from build123d import *

# Parameters (mm, degrees)
CROQUIS1_W              = 44
CROQUIS1_H              = 20
CROQUIS1_R              = 8
SALIENTE_EXTRUIR1_DEPTH = 15
CROQUIS2_R              = 1.75
CORTAR_EXTRUIR1_DEPTH   = 22


with BuildPart() as part:
    # Croquis1 → Saliente-Extruir1 (new body)
    with BuildSketch(Plane.XY):
        Rectangle(CROQUIS1_W, CROQUIS1_H)
        with Locations((-11, 0)):
            Circle(CROQUIS1_R, mode=Mode.SUBTRACT)
        with Locations((11, 0)):
            Circle(CROQUIS1_R, mode=Mode.SUBTRACT)
    extrude(amount=SALIENTE_EXTRUIR1_DEPTH)

    # Croquis2 → Cortar-Extruir1 (cut)
    with BuildSketch(Plane.XY.offset(15)):
        with Locations((-19, 7)):
            Circle(CROQUIS2_R)
        with Locations((19, -7)):
            Circle(CROQUIS2_R)
        with Locations((19, 7)):
            Circle(CROQUIS2_R)
        with Locations((-19, -7)):
            Circle(CROQUIS2_R)
    extrude(amount=-CORTAR_EXTRUIR1_DEPTH, mode=Mode.SUBTRACT)


solid = part.part
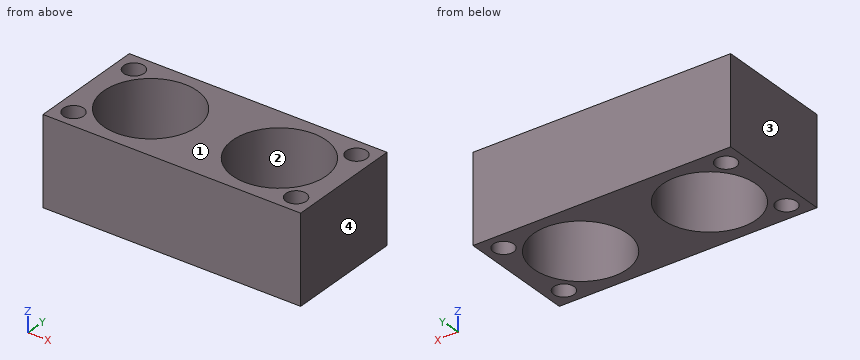
Here's how the part is built. I have some questions about the finished solid (model axes, mm). Face numbers are marked on the shaded views. Coordinates: 2 decimals unless noted, no trailing zeros. Write each loop counter-clockwise with the first axis right and the second up, starting at its lowest first coordinate (ties: lowest second). Pieces come first, ordered by that corner, then holes.
1) If we section it at D-D (y = 7): List the corners of the cut face in (x, z) for me.
Filled in:
outline: (-22, 0) - (-20.75, 0) - (-20.75, 15) - (-22, 15) - close; (-17.25, 0) - (-14.87, 0) - (-14.87, 15) - (-17.25, 15) - close; (-7.13, 0) - (7.13, 0) - (7.13, 15) - (-7.13, 15) - close; (14.87, 0) - (17.25, 0) - (17.25, 15) - (14.87, 15) - close; (20.75, 0) - (22, 0) - (22, 15) - (20.75, 15) - close
2) Thinking about a two-plate mould opening in X: for the marked faces 1, 2, 3 and 4, which applies, +X half, -X half, draft (parallel to the pull), parting line (faces both ways), or undercut?
Filled in:
face 1: draft
face 2: undercut
face 3: -X half
face 4: +X half
3) If we section it at A-A (z = 12.5): List the corners of the cut face in (x, y) for me, plus the area to 3 significant figures.
Filled in:
outline: (-22, -10) - (22, -10) - (22, 10) - (-22, 10) - close; hole circle Ø3.5 at (-19, -7); hole circle Ø3.5 at (-19, 7); hole circle Ø16 at (-11, 0); hole circle Ø16 at (11, 0); hole circle Ø3.5 at (19, -7); hole circle Ø3.5 at (19, 7)
area: 439 mm2
4) If I drill on line 1 (Y direction, x = -11, z = 10.5); line 2 (X direction, y = 4.25, z = 10.5); line 3 (X direction, y = -4.75, z = 2), over which ranges is the centre line in solid material (lowest first)?
Filled in:
line 1: y = -10 to -8, 8 to 10
line 2: x = -22 to -17.78, -4.22 to 4.22, 17.78 to 22
line 3: x = -22 to -17.44, -4.56 to 4.56, 17.44 to 22
5) If we section it at C-C (x = -11): List the corners of the cut face in (y, z) for me, plus the area to 3 significant figures.
Filled in:
outline: (-10, 0) - (-8, 0) - (-8, 15) - (-10, 15) - close; (8, 0) - (10, 0) - (10, 15) - (8, 15) - close
area: 60.0 mm2
6) If we section it at B-B (y = 0): List the corners of the cut face in (x, z) for me.
Filled in:
outline: (-22, 0) - (-19, 0) - (-19, 15) - (-22, 15) - close; (-3, 0) - (3, 0) - (3, 15) - (-3, 15) - close; (19, 0) - (22, 0) - (22, 15) - (19, 15) - close
